The listing builds one solid part. Answer for the finished solid, in the listing's coordinates (mm). A direction names the side the tool comes from. Round coordinates to 2 decimals unless told otherwise and drop trailing zeros. Write each loop counter-clockwise with the first axis right and the second up, starting at its lowest first coordinate (ties: lowest second). Pieces come first, ordered by that corner, then holes. Notation, with made-up numbers: M 73.5,-33.75 L 125.5,-33.75 A31 cw 125.5,-3.75 Z; hole C 39,-15 d11. An arc over 180 degrees is marked long. Write each question's results on one line, items separated by ' | '.
from build123d import *

# Parameters (mm, degrees)
SKETCH1_R           = 3.875
BOSS_EXTRUDE1_DEPTH = 4.75
FILLET1_R           = 0.25
CUT_EXTRUDE1_DEPTH  = 2.75
SKETCH3_R           = 2.375
BOSS_EXTRUDE2_DEPTH = 10


with BuildPart() as part:
    # Sketch1 → Boss-Extrude1 (new body)
    with BuildSketch(Plane(origin=(0, 0, 0), x_dir=(1, 0, 0), z_dir=(0, 1, 0))):
        Circle(SKETCH1_R)
    extrude(amount=BOSS_EXTRUDE1_DEPTH)

    # Fillet1
    fillet1_edges = [part.edges().sort_by_distance(p)[0] for p in [
        (-3.875, 4.75, 0),
    ]]
    fillet(fillet1_edges, radius=FILLET1_R)

    # Sketch2 → Cut-Extrude1 (cut)
    with BuildSketch(Plane(origin=(0, 4.75, 0), x_dir=(1, 0, 0), z_dir=(0, 1, 0))):
        Polygon((-2.424871131, 0), (-1.212435565, -2.1), (1.212435565, -2.1), (2.424871131, 0), (1.212435565, 2.1), (-1.212435565, 2.1), align=None)
    extrude(amount=-CUT_EXTRUDE1_DEPTH, mode=Mode.SUBTRACT)

    # Sketch3 → Boss-Extrude2 (add)
    with BuildSketch(Plane.XZ):
        Circle(SKETCH3_R)
    extrude(amount=BOSS_EXTRUDE2_DEPTH)

    # Sketch4 → Cut-Revolve1 (revolve, cut)
    with BuildSketch(Plane(origin=(0, 0, 0), x_dir=(0, 0, -1), z_dir=(1, 0, 0))):
        Polygon((-2.375, -10), (-2.375, -9.375), (-1.75, -10), align=None)
    revolve(axis=Axis((0, -10, 0), (0, 1, 0)), mode=Mode.SUBTRACT)


solid = part.part
1) Section A-A (y = 3.25) is taken. Determine the outline of the cut face in (x, z) (3 decimals), then the cut area to 3 significant figures.
Return value:
outline: C 0,0 d7.75; hole M -2.425,0 L -1.212,-2.1 L 1.212,-2.1 L 2.425,0 L 1.212,2.1 L -1.212,2.1 Z | area: 31.9 mm²
2) Each of these flat-tipped pins is pushed along its axis until it touches: pin 1 (1 mm diameter, centred on y = -8, z = -2.5, fed in from +X); pin 2 (1 mm diameter, centred on y = -3, z = -1, fed in from -X); pin 3 (1.5 mm diameter, centred on x = 3, z = 2, fed in from -Y). Where does it stop, or does it pass through?
Return value:
pin 1: x = 1.28 | pin 2: x = -2.32 | pin 3: y = 0
3) Find the intervals of material crossed by line 1 (Z direction, x = 0, y = 3) (3 decimals); line 2 (Y direction, x = 3.5, z = 0.5); line 3 (Y direction, x = 1.5, z = 0), in increasing order.
Return value:
line 1: -3.875 to -2.1, 2.1 to 3.875 | line 2: 0 to 4.75 | line 3: -10 to 2
4) Section C-C (y = -7) is taken. Determine the outline of the cut face in (x, z) (3 decimals), then the cut area to 3 significant figures.
Return value:
outline: C 0,0 d4.75 | area: 17.7 mm²
5) Section D-D (y = 1.5) is taken. Determine the outline of the cut face in (x, z) (3 decimals).
Return value:
outline: C 0,0 d7.75
6) A tool of negligible diameter and unlimited length cuts with its end or side. For faces 4 (the face through (0, 3, -2.1)), 5 (the face through (0, -10, 0)), from which of +Z, -Z, +X, -X, +Y, -Y can it reach the whole face along a straight path? Write none if from no direction.
Return value:
face 4: +Y | face 5: +Z, -Z, +X, -X, -Y
7) The mould has two halves that part along Z. Classify faces 1 (the face through (-2, 0, 2)), 2 (the face through (2.265, -4.622, 0.713)), 3 (the face through (-1.81, 3.394, -1.065)): +Z half, -Z half, draft (parallel to the pull), parting line (faces both ways), or undercut.
Return value:
face 1: draft | face 2: parting line | face 3: undercut
8) Section B-B (x = 0) is taken. Determine the outline of the cut face in (y, z) (3 decimals).
Return value:
outline: M -10,-1.75 L -9.375,-2.375 L 0,-2.375 L 0,-3.875 L 4.5,-3.875 A0.25 ccw 4.75,-3.625 L 4.75,-2.1 L 2,-2.1 L 2,2.1 L 4.75,2.1 L 4.75,3.625 A0.25 ccw 4.5,3.875 L 0,3.875 L 0,2.375 L -9.375,2.375 L -10,1.75 Z
